from build123d import *

# Parameters (mm, degrees)
F0_W     = 273.05
F0_H     = 76.2
F1_DEPTH = 6.35
F2_W     = 6.35
F2_H     = 15.875
F2_H_2   = 9.525
F3_DEPTH = 6.35
F4_W     = 25.4
F4_H     = 6.35
F5_DEPTH = 6.351
F6_W     = 6.35
F6_H     = 9.525
F7_DEPTH = 6.35


with BuildPart() as f1:
    # F0 (on Front) → F1 (new body)
    with BuildSketch(Plane.XZ):
        with Locations((136.525, 38.1)):
            Rectangle(F0_W, F0_H)
    extrude(amount=F1_DEPTH)

    # F2 (on face) → F3 (cut, through all)
    with BuildSketch(Plane.XZ.offset(6.35)):
        with Locations((3.175, 58.7375)):
            Rectangle(F2_W, F2_H)
        with Locations((3.175, 33.3375)):
            Rectangle(F2_W, F2_H)
        with Locations((3.175, 11.1125)):
            Rectangle(F2_W, F2_H_2)
        with Locations((269.875, 11.1125)):
            Rectangle(F2_W, F2_H_2)
        with Locations((269.875, 33.3375)):
            Rectangle(F2_W, F2_H)
        with Locations((269.875, 58.7375)):
            Rectangle(F2_W, F2_H)
    extrude(amount=-F3_DEPTH, mode=Mode.SUBTRACT)

    # F4 (on face) → F5 (cut, through all)
    with BuildSketch(Plane.XZ.offset(6.35)):
        with Locations((12.7, 3.175)):
            Rectangle(F4_W, F4_H)
        with Locations((63.5, 3.175)):
            Rectangle(F4_W, F4_H)
        with Locations((114.3, 3.175)):
            Rectangle(F4_W, F4_H)
        with Locations((165.1, 3.175)):
            Rectangle(F4_W, F4_H)
        with Locations((215.9, 3.175)):
            Rectangle(F4_W, F4_H)
        with Locations((266.7, 3.175)):
            Rectangle(F4_W, F4_H)
    extrude(amount=-F5_DEPTH, mode=Mode.SUBTRACT)

    # F6 (on face) → F7 (cut, through all)
    with BuildSketch(Plane.XZ.offset(6.35)):
        with Locations((269.875, 46.0375)):
            Rectangle(F6_W, F6_H)
    extrude(amount=-F7_DEPTH, mode=Mode.SUBTRACT)


solid = f1.part
The listing builds one solid part. Answer for the finished solid, in the listing's coordinates (mm). A direction names the side the tool comes from. Round coordinates to 2 decimals unless told otherwise and drop trailing zeros. Write each loop counter-clockwise with the first axis right and the second up, starting at its lowest first coordinate (ties: lowest second). Pieces come first, ordered by that corner, then holes. Notation, with made-up numbers: M -26.5,39.25 L -21.5,39.25 A12 ccw -21.5,47.25 Z; hole C 26,-13.5 d8. An arc over 180 degrees is marked long. Write each question's results on one line, items separated by ' | '. Start each with the question number.
Item 1: For faces 5 (the face through (50.8, -3, 3)), 6 (the face through (16, -3, 6.35)), 7 (the face through (6.35, -3, 33)), determine the directions among +Z, -Z, +X, -X, +Y, -Y from which every point of the face is accessible in a straight line to the end or side of a thin tool.
Item 2: Flat-ended cylindrical pins translate along their axes: pin 1 Ø1.9 at (y, z) = (-4.5, 2.5) entering from -X; pin 2 Ø3 at (x, y) = (166.5, -4.5) entering from -Z; pin 3 Ø3 at (y, z) = (-2, 2) entering from +X. Find the tip coordinate at first contact, or state that the pin passes through.
Item 3: For a pull along X with two mould halves and no side action, classify faces 1 (the face through (3, -3, 50.8)), 2 (the face through (266.7, -3, 46)), 3 (the face through (127, -3, 3)), 4 (the face through (0, -3, 21)) as pulls with the +X half, pulls with the -X half, needs draft (parallel to the pull), parting line crosses it, or undercut.
Item 4: A cutting plane is placed at B-B on x = 54. Write down the section's boundary in (y, z), and give its area (3 significant figures).
Item 5: A cutting plane is placed at A-A on z = 10. Write down the section's boundary in (x, y), and give its area (3 significant figures).
Item 6: Straight lines are drawn through the part: L1, parallel to X at y = -2.5, z = 34; L2, parallel to X at y = -2, z = 44.5; L3, parallel to Z at x = 208.5, y = -1. For each, find the intervals that lie inside material, in ascending order. Write a range as [from, to].
Check sheet entries:
1) face 5: -Z, +Y, -Y | face 6: -Z, -X, +Y, -Y | face 7: -X, +Y, -Y
2) pin 1: x = 25.4 | pin 2: z = 6.35 | pin 3: x = 254
3) face 1: needs draft | face 2: pulls with the +X half | face 3: undercut | face 4: pulls with the -X half
4) outline: M -6.35,6.35 L 0,6.35 L 0,76.2 L -6.35,76.2 Z | area: 444 mm²
5) outline: M 6.35,-6.35 L 266.7,-6.35 L 266.7,0 L 6.35,0 Z | area: 1,650 mm²
6) L1: [6.35, 266.7] | L2: [0, 266.7] | L3: [6.35, 76.2]
